Autodesk Inventor part; units mm, degrees
ref_plane "YZ Plane" through (0, 0, 0) normal (1, 0, 0) x (0, 1, 0)
ref_plane "XZ Plane" through (0, 0, 0) normal (0, 1, 0) x (-1, 0, 0)
ref_plane "XY Plane" through (0, 0, 0) normal (0, 0, 1) x (1, 0, 0)
sketch "Sketch1" plane through (0, 0, 0) normal (1, 0, 0) x (0, 1, 0)
  point P0 (0, 0)
sketch "Sketch2" plane through (0, 0, 0) normal (1, 0, 0) x (0, 1, 0)
  line L0 (7.3233, 8.5443) -> (7.3233, 8.5443)
  line L1 (4.1483, 5.3693) -> (-70.0914, 5.3693)
  line L2 (4.1483, 11.7193) -> (-63.7414, 11.7193)
  line L3 (-70.0914, 60.6498) -> (-70.0914, 5.3693)
  line L4 (7.3233, 103.7583) -> (7.3233, 103.7583)
  line L5 (-63.7414, 62.4452) -> (-63.7414, 11.7193)
  arc A0 (7.3233, 8.5443) -> (4.1483, 11.7193) centre (4.1483, 8.5443) ccw
  arc A1 (4.1483, 5.3693) -> (7.3233, 8.5443) centre (4.1483, 8.5443) ccw
  line L6 (-70.0914, 60.6498) -> (-70.0914, 119.6333)
  line L7 (-70.0914, 119.6333) -> (4.1483, 119.6333)
  line L8 (-63.7414, 62.4452) -> (-63.7414, 113.2833)
  line L9 (-63.7414, 113.2833) -> (13.8631, 113.2833)
  line L10 (4.1483, 119.6333) -> (4.1483, 119.6333)
  line L11 (7.3233, 116.4583) -> (7.3233, 116.4583)
  arc A2 (7.3233, 116.4583) -> (4.1483, 119.6333) centre (4.1483, 116.4583) ccw
  arc A3 (4.1483, 113.2833) -> (7.3233, 116.4583) centre (4.1483, 116.4583) ccw
  point P0 (0, 0)
  point P1 (7.3233, 11.7193)
  point P2 (7.3233, 5.3693)
  point P3 (7.3233, 106.9333)
  point P4 (7.3233, 100.5833)
  point P5 (7.3233, 8.5443)
  point P6 (7.3233, 119.6333)
  point P7 (4.1483, 113.2833)
  point P8 (4.1483, 119.6333)
  dimension "d0" = 6.35
  dimension "d35" = 3.175
  dimension "d36" = 3.175
  dimension "d42" = 6.35
  dimension "d43" = 6.35
extrude "Extrusion1" add sketch "Sketch2" along normal blind 25.4
sketch "Sketch4" plane through (0, -70.0914, 5.3693) normal (0, -1, 0) x (1, 0, 0)
  line L0 (0, 0) -> (25.4, 0)
  line L1 (25.4, 114.264) -> (25.4, 0)
  line L2 (25.4, 57.132) -> (12.7, 57.132)
  line L3 (19.05, 44.432) -> (6.35, 44.432)
  line L4 (6.35, 44.432) -> (6.35, 69.832)
  line L5 (6.35, 69.832) -> (19.05, 69.832)
  line L6 (19.05, 69.832) -> (19.05, 44.432)
  line L7 (19.05, 44.432) -> (6.35, 69.832) construction
  line L8 (6.35, 44.432) -> (19.05, 69.832) construction
  point P0 (0, -5.3693)
  point P1 (25.4, 101.6762)
  dimension "d48" = 12.7
  dimension "d49" = 25.4
sketch "Sketch6" plane through (0, -70.0914, 119.6333) normal (0, 0, 1) x (1, 0, 0)
  line L0 (0, 77.4147) -> (25.4, 77.4147)
  line L1 (0, 77.4147) -> (25.4, 77.4147)
  circle A0 centre (12.7, 71.0647) radius 0.9144
  point P0 (0, 70.0914)
  dimension "d45" = 1.8288
extrude "Extrusion6" cut sketch "Sketch6" against normal through all
extrude "Extrusion7" cut sketch "Sketch4" against normal through all
sketch "Sketch7" plane through (0, -70.0914, 5.3693) normal (0, -1, 0) x (1, 0, 0)
  line L0 (19.05, 69.832) -> (6.35, 69.832)
  line L1 (6.35, 44.432) -> (19.05, 44.432)
  circle A0 centre (12.7, 71.356) radius 1.0033
  circle A1 centre (12.7, 42.908) radius 1.0033
  point P0 (0, -5.3693)
  dimension "d55" = 2.0066
extrude "Extrusion8" cut sketch "Sketch7" against normal through all
properties part number "1st Servo Holder"
Geometry check sheet. Reference: the model listing, model coordinates, mm. A direction names the side the tool comes from. Round coordinates to 2 decimals unless told otherwise and drop trailing zeros. Write each loop counter-clockwise with the first axis right and the second up, starting at its lowest first coordinate (ties: lowest second). Pieces come first, ordered by that corner, then holes. Notation, with made-up numbers: (61, 85) - (106, 85) arc R19 cw to (106, 106) - close; hole circle Ø6 at (10.5, 88.5). An arc over 180 degrees is marked (long way). One line per item, written item: value.
1. Scan lines: L1, parallel to Z at x = 12.7, y = -66; L2, parallel to Z at x = 15.5, y = -29.5; L3, parallel to Y at x = 18.25, z = 84. Record each from-to range of solid material in increasing order.
The answers:
L1: z = 5.37 to 47.27, 49.28 to 49.8, 75.2 to 75.72, 77.73 to 119.63
L2: z = 5.37 to 11.72, 113.28 to 119.63
L3: y = -70.09 to -63.74
2. Cross-section at A-A on z = 64. Record the boundary of the cut face in (x, y).
The answers:
outline: (0, -70.09) - (6.35, -70.09) - (6.35, -63.74) - (0, -63.74) - close; (19.05, -70.09) - (25.4, -70.09) - (25.4, -63.74) - (19.05, -63.74) - close
3. Cross-section at C-C on x = 16.75. Record the boundary of the cut face in (y, z) (3 decimals), and give its area (3 significant figures).
The answers:
outline: (-70.091, 5.369) - (4.148, 5.369) arc R3.175 ccw to (4.148, 11.719) - (-63.741, 11.719) - (-63.741, 49.801) - (-70.091, 49.801) - close; (-70.091, 75.201) - (-63.741, 75.201) - (-63.741, 113.283) - (4.148, 113.283) arc R3.175 ccw to (4.148, 119.633) - (-70.091, 119.633) - close
area: 1,460 mm^2
4. Set-up check for faces 1 (the face through (19.05, -67, 63)), 2 (the face through (13, -32, 5.369)), 3 (the face through (13, -30, 113.283)): record each of +Z, -Z, +X, -X, +Y, -Y from which the full face is reachable in a straight line by a thin tool's end or side.
The answers:
face 1: +Y, -Y
face 2: -Z, +X, -X, +Y, -Y
face 3: +X, -X, +Y
5. Cross-section at D-D on x = 5. Record the boundary of the cut face in (y, z) (3 decimals).
The answers:
outline: (-70.091, 5.369) - (4.148, 5.369) arc R3.175 ccw to (4.148, 11.719) - (-63.741, 11.719) - (-63.741, 113.283) - (4.148, 113.283) arc R3.175 ccw to (4.148, 119.633) - (-70.091, 119.633) - close
6. Depth check by flat-ended pin: pin 1 Ø1.8 at (x, z) = (12.7, 48.28) entering from +Y; pin 2 Ø12.5 at (x, z) = (13.5, 50) entering from +Y. Enter the tip coordinate at first touch or a pass-through.
The answers:
pin 1: passes through
pin 2: stops at y = -63.74
7. Mould release check, pull along X, two halves, no side actions. Record for faces 4 (the face through (6.35, -67, 62)), 5 (the face through (13, -67, 75.201)), 6 (the face through (13, -33, 119.633)), 7 (the face through (0, -66, 71)): released by +X, released by -X, zero draft, split by the parting line, or undercut.
The answers:
face 4: undercut
face 5: undercut
face 6: zero draft
face 7: released by -X
8. Cross-section at B-B on y = -23. Record the boundary of the cut face in (x, z), and give its area (3 significant figures).
The answers:
outline: (0, 5.37) - (25.4, 5.37) - (25.4, 11.72) - (0, 11.72) - close; (0, 113.28) - (25.4, 113.28) - (25.4, 119.63) - (0, 119.63) - close
area: 323 mm^2
